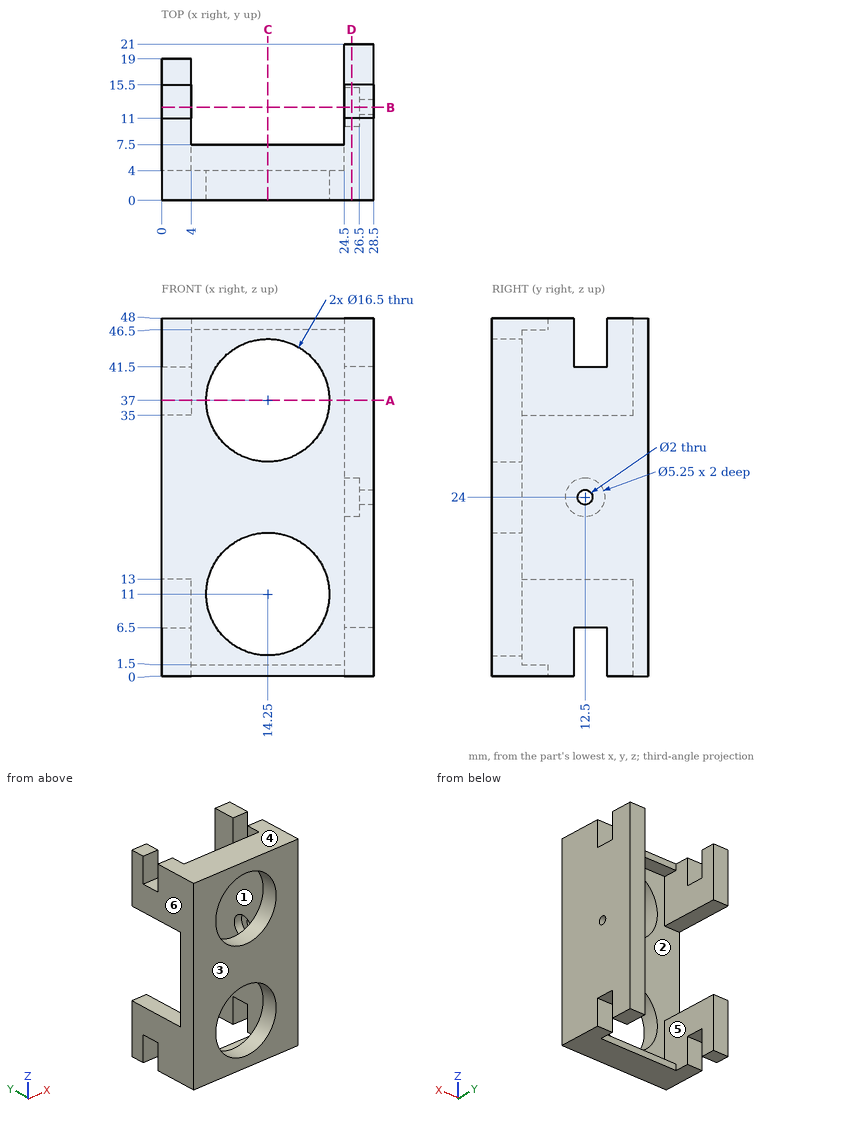
Design review of the part shown in the three views and the two pictorial views. Dimensions are in mm from the part's minimum x, y and z. A direction names the side the tool comes from. Coordinates: 2 decimals unless noted, no trailing zeros. Loops run counter-clockwise (first coordinate to the right, second up) from the corner with the lowest first, then second, coordinate; pieces in that order, holes last. Notation, with made-up numbers: M 22,16 L 36,16 A15 cw 36,29 Z; hole C 33.5,87 d10. An arc over 180 degrees is marked long. Put each result on its own line as item: value. Start each with the question number.
Q1. Add section A-A (z = 37). Write out the cut boundary in (x, y).
Q2. The part is to be moulded in two halves that separate along Z. For the marked faces 1, 2, 3 and 4, say which applies: +Z half, -Z half, draft (parallel to the pull), parting line (faces both ways), or undercut.
Q3. Clearance check with flat-ended pins moving along their axes: pin 1 (3 mm diameter, centred on x = 10.5, z = 29.5, fed in from +Y); pin 2 (12 mm diameter, centred on y = 5, z = 30, fed in from -X); pin 3 (2 mm diameter, centred on x = 1, z = 4, fed in from +Y); pin 4 (3 mm diameter, centred on y = 12.5, z = 24, fed in from -X). State where each tip first meets the part, or that it passes through.
Q4. Add section D-D (x = 25.5). Write out the cut boundary in (y, z) (3 decimals).
Q5. For the marked faces 5 and 6, list the 3-axis set-ups (+Z, -Z, +X, -X, +Y, -Y) from which the entire face can be reached by the end or side of a thin tool; tool diameter is ignored.
Q6. Wall thickness on line 1 (Z direction, x = 14.25, y = 1.6); line 2 (X direction, y = 18.5, z = 39); line 3 (Y direction, x = 25.9, z = 24) (3 decimals): over which ranges is each line inside the solid? List them lowest first.
Q7. Add section C-C (x = 14.25). Write out the cut boundary in (y, z), and give its area (3 significant figures).
Q8. Add section B-B (y = 12.5). Write out the cut boundary in (x, z) (3 decimals).
Answers:
1. outline: M 0,0 L 6,0 L 6,4 L 4,4 L 4,19 L 0,19 Z; M 22.5,0 L 28.5,0 L 28.5,21 L 24.5,21 L 24.5,4 L 22.5,4 Z
2. face 1: undercut
2. face 2: undercut
2. face 3: draft
2. face 4: +Z half
3. pin 1: stops at y = 4
3. pin 2: stops at x = 0
3. pin 3: stops at y = 19
3. pin 4: stops at x = 26.5
4. outline: M 0,0 L 11,0 L 11,6.5 L 15.5,6.5 L 15.5,0 L 21,0 L 21,48 L 15.5,48 L 15.5,41.5 L 11,41.5 L 11,48 L 0,48 Z; hole C 12.5,24 d5.25
5. face 5: +Y
5. face 6: +Z, -Z, -X, +Y, -Y
6. line 1: z = 0 to 2.75, 19.25 to 28.75, 45.25 to 48
6. line 2: x = 0 to 4, 24.5 to 28.5
6. line 3: y = 0 to 9.875, 15.125 to 21
7. outline: M 0,0 L 7.5,0 L 7.5,1.5 L 4,1.5 L 4,2.75 L 0,2.75 Z; M 0,19.25 L 4,19.25 L 4,28.75 L 0,28.75 Z; M 0,45.25 L 4,45.25 L 4,46.5 L 7.5,46.5 L 7.5,48 L 0,48 Z
7. area: 70.5 mm^2
8. outline: M 0,6.5 L 4,6.5 L 4,13 L 0,13 Z; M 0,35 L 4,35 L 4,41.5 L 0,41.5 Z; M 24.5,6.5 L 28.5,6.5 L 28.5,23 L 26.5,23 L 26.5,21.375 L 24.5,21.375 Z; M 24.5,26.625 L 26.5,26.625 L 26.5,25 L 28.5,25 L 28.5,41.5 L 24.5,41.5 Z
